```python
from build123d import *

# Parameters (mm, degrees)
F0_W     = 104.369306
F0_H     = 129.608706
F1_DEPTH = 214.884
F2_W     = 99.349372
F2_H     = 104.369306
F3_DEPTH = 116.078
F4_W     = 99.349372
F4_H     = 129.608706
F5_DEPTH = 96.774
F6_R     = 13.7414
F7_DEPTH = 25.4


with BuildPart() as f1:
    # F0 (on Right) → F1 (new body)
    with BuildSketch(Plane.YZ):
        Rectangle(F0_W, F0_H)
    extrude(amount=F1_DEPTH)

    # F2 (on face) → F3 (join)
    with BuildSketch(Plane.XY.offset(64.804353)):
        with Locations((49.674686, 0)):
            Rectangle(F2_W, F2_H)
    extrude(amount=F3_DEPTH)

    # F4 (on face) → F5 (join)
    with BuildSketch(Plane(origin=(0, 52.184653, 0), x_dir=(-1, 0, 0), z_dir=(0, 1, 0))):
        with Locations((-49.674686, 0)):
            Rectangle(F4_W, F4_H)
    extrude(amount=F5_DEPTH)

    # F6 (on face) → F7 (cut)
    with BuildSketch(Plane(origin=(0, 0, -64.804353), x_dir=(1, 0, 0), z_dir=(0, 0, -1))):
        with Locations((19.05245, 32.441348)):
            Circle(F6_R)
    extrude(amount=-F7_DEPTH, mode=Mode.SUBTRACT)


solid = f1.part
```
Here's how the part is built. I have some questions about the finished solid (model axes, mm). A direction names the side the tool comes from. Give positions to 0.01 mm unless a question says otherwise; leave off trailing zeros. Order: outer loops, then holes, each group sorted by start corner. A loop starts at its lowest first (then second) coordinate and runs counter-clockwise, first axis right, second up. Notation, with made-up numbers: M 24,47.5 L 56,47.5 A26 cw 56,81.5 Z; hole C -33,29.25 d3. An arc over 180 degrees is marked long. Use a Markdown table: item, result. Add a question column.
1. Suppose I cut it at D-D (x = 104). List the corners of the cut face in (y, z) for me.
2. If we mould it in two halves opening along Y, with no side actions, what happens to faces 4 (the flat face through (19, -33, -39.404)), 5 (the flat face through (156, -1, 64.804)), 6 (the flat face through (156, 52.185, -1))? For each: +Y half, -Y half, draft (parallel to the pull), parting line (faces both ways), or undercut.
3. Suppose I cut it at B-B (y = 47). List the corners of the cut face in (x, z) for me, and give its area (3 significant figures).
4. On a 3-axis mill with a long thin cutter (end or side, diameter ignored), from which of +Z, -Z, +X, -X, +Y, -Y can I reach the whole of each face in a straight line? I mean faces 1 (the cylindrical face through (8.9, -41.7, -52.3)), 2 (the flat face through (99.349, -1, 122)), 3 (the flat face through (49, 52.185, 122)). Say none if no direction works.
5. I need wall thicknesses on probe 1 along Z at (x, y) = (180, 15); probe 2 along Y at (x, z) = (198, -42.5); probe 3 along X at (y, z) = (9.5, 75.5). Which ranges of each line are inside material? Lowest first, please. Write a range as from..to.
6. Suppose I cut it at C-C (z = -47.5). List the corners of the cut face in (x, y) for me.
7. For pin 1 Ø16.5 at (x, y) = (19.05, -32.44) entering from -Z; pin 2 Ø6 at (y, z) = (98.5, 13) entering from +X, each with a flat end and sliding along its axis, tell me the tip position at first contact or that it passes through.
8. Suppose I cut it at A-A (z = 0.5). List the corners of the cut face in (x, y) for me.
Results list:
| question | item | result |
|---|---|---|
| 1 | outline | M -52.18,-64.8 L 52.18,-64.8 L 52.18,64.8 L -52.18,64.8 Z |
| 2 | face 4 | undercut |
| 2 | face 5 | draft |
| 2 | face 6 | +Y half |
| 3 | outline | M 0,-64.8 L 214.88,-64.8 L 214.88,64.8 L 99.35,64.8 L 99.35,180.88 L 0,180.88 Z |
| 3 | area | 39,400 mm² |
| 4 | face 1 | -Z |
| 4 | face 2 | +Z, +X, +Y, -Y |
| 4 | face 3 | +Z, +X, -X, +Y |
| 5 | probe 1 | z = -64.8..64.8 |
| 5 | probe 2 | y = -52.18..52.18 |
| 5 | probe 3 | x = 0..99.35 |
| 6 | outline | M 0,-52.18 L 214.88,-52.18 L 214.88,52.18 L 99.35,52.18 L 99.35,148.96 L 0,148.96 Z; hole C 19.05,-32.44 d27.48 |
| 7 | pin 1 | stops at z = -39.4 |
| 7 | pin 2 | stops at x = 99.35 |
| 8 | outline | M 0,-52.18 L 214.88,-52.18 L 214.88,52.18 L 99.35,52.18 L 99.35,148.96 L 0,148.96 Z |
